```python
from build123d import *

# Parameters (mm, degrees)
F_6_0_6_DIAMETER_HOLE2_D     = 6
F_6_0_6_DIAMETER_HOLE2_DEPTH = 24
F_6_0_6_DIAMETER_HOLE2_TIP   = 1.802581857


with BuildPart() as part:
    # Sketch1 → Revolve1 (revolve)
    with BuildSketch(Plane(origin=(0, 0, 0), x_dir=(1, 0, 0), z_dir=(0, 1, 0))):
        Polygon((0, -11.46), (-5.15, -11.46), (-5.15, -13), (-7, -13), (-7, 0), (7, 0), (7, -13), (5.15, -13), (5.15, -11.46), align=None)
    revolve(axis=Axis((-7, 0, 0), (1, 0, 0)))

    # Ø6.0 (6) Diameter Hole2
    with Locations(Plane(origin=(7, 0, 0), x_dir=(0, 0, -1), z_dir=(1, 0, 0))):
        with Locations((0, 0)):
            Hole(F_6_0_6_DIAMETER_HOLE2_D / 2, depth=F_6_0_6_DIAMETER_HOLE2_DEPTH)
            with Locations((0, 0, -(F_6_0_6_DIAMETER_HOLE2_DEPTH + F_6_0_6_DIAMETER_HOLE2_TIP / 2))):  # 118° drill point
                Cone(0, F_6_0_6_DIAMETER_HOLE2_D / 2, F_6_0_6_DIAMETER_HOLE2_TIP, mode=Mode.SUBTRACT)


solid = part.part
```
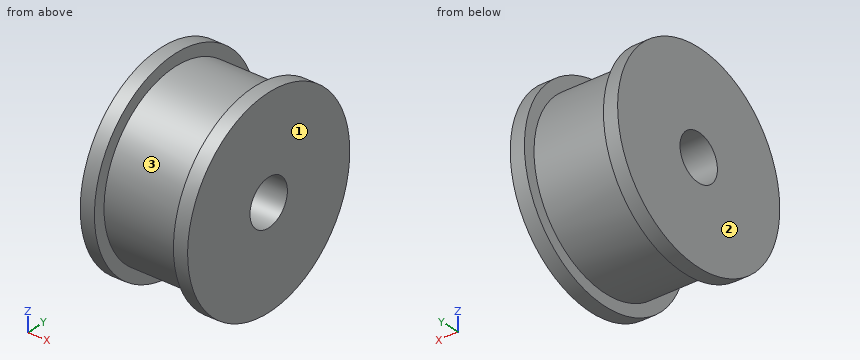
Design review of the part built by this model. Coordinates are the model's own, in mm. Face numbers are marked on the shaded views. Coordinates: 2 decimals unless noted, no trailing zeros. Order: outer loops, then holes, each group sorted by start corner. A loop starts at its lowest first (then second) coordinate and runs counter-clockwise, first axis right, second up. Notation, with made-up numbers: (39.5, -10.5) -> (53.5, -10.5) arc R21 ccw to (53.5, -4.5) -> close; hole circle Ø4 at (33.25, 17). An arc over 180 degrees is marked (long way). One line per item, written item: value. Start each with the question number.
Q1. Take a section at A-A, the plane z = 0. State the section outline as (x, y) points.
Q2. Insertion check: pin 1 Ø2 at (x, z) = (-5.5, 7.5) entering from +Y; pin 2 Ø8 at (x, z) = (5.5, 7.5) entering from +Y; pin 3 Ø1 at (x, z) = (-1, -0.5) entering from +Y. Each pin has a flat end and moves straight along its axis. Give the tip position at first contact, or say it passes through.
Q3. Mouldability with a two-part tool opening along X and no side actions: class the marked faces 1, 2 and 3 as pulls with the +X half, pulls with the -X half, needs draft (parallel to the pull), parting line crosses it, or undercut.
Q4. For probe 1 along X at (y, z) = (11.75, -2.25); probe 2 along Y at (x, z) = (-3, 0); probe 3 along Z at (x, y) = (-0.5, -2), list the stretches that pass through material, from the lowest coordinate up.
Q5. Take a section at C-C, the plane x = -5.75. State the section outline as (y, z) points, then the cut area to 3 significant figures.
Q6. Take a section at D-D, the plane y = 4. State the section outline as (x, z) points.
Values follow:
1. outline: (-7, -13) -> (-5.15, -13) -> (-5.15, -11.46) -> (5.15, -11.46) -> (5.15, -13) -> (7, -13) -> (7, -3) -> (-7, -3) -> close; (-7, 3) -> (7, 3) -> (7, 13) -> (5.15, 13) -> (5.15, 11.46) -> (-5.15, 11.46) -> (-5.15, 13) -> (-7, 13) -> close
2. pin 1: stops at y = 11.26
2. pin 2: stops at y = 12.52
2. pin 3: stops at y = 11.46
3. face 1: pulls with the +X half
3. face 2: pulls with the -X half
3. face 3: undercut
4. probe 1: x = -7 to -5.15, 5.15 to 7
4. probe 2: y = -11.46 to -3, 3 to 11.46
4. probe 3: z = -11.28 to -2.24, 2.24 to 11.28
5. outline: circle Ø26 at (0, 0); hole circle Ø6 at (0, 0)
5. area: 503 mm2
6. outline: (-7, -12.37) -> (-5.15, -12.37) -> (-5.15, -10.74) -> (5.15, -10.74) -> (5.15, -12.37) -> (7, -12.37) -> (7, 12.37) -> (5.15, 12.37) -> (5.15, 10.74) -> (-5.15, 10.74) -> (-5.15, 12.37) -> (-7, 12.37) -> close
